from build123d import *

# Parameters (mm, degrees)
F0_W      = 59.0042
F0_H      = 41.021
F1_DEPTH  = 13.97
F2_R      = 2.54
F3_W      = 36.449
F3_H      = 36.449
F4_DEPTH  = 11.43
F5_W      = 25.146
F5_H      = 25.146
F6_DEPTH  = 2.541
F7_R      = 1.5875
F8_DEPTH  = 12.7
F9_W      = 9.144
F9_H      = 13.97
F10_DEPTH = 25.019
F11_R     = 6.98499
F12_W     = 3.3528
F12_H     = 22.225
F13_DEPTH = 13.971
F14_R     = 2.54
F15_DEPTH = 34.0878


# Not quite as in the source:
# - a fillet or chamfer is up to 0.001 mm smaller than in the source, because OpenCascade refuses the exact size


with BuildPart() as f1:
    # F0 (on Top) → F1 (new body)
    with BuildSketch(Plane.XY):
        with Locations((4.1021, 4.8895)):
            Rectangle(F0_W, F0_H)
    extrude(amount=F1_DEPTH)

    # F2
    f2_edges = [f1.edges().sort_by_distance(p)[0] for p in [
        (-25.4, 25.4, 6.985),
        (33.6042, 25.4, 6.985),
        (33.6042, -15.621, 6.985),
        (-25.4, -15.621, 6.985),
    ]]
    fillet(f2_edges, radius=F2_R)

    # F3 (on face) → F4 (cut)
    with BuildSketch(Plane.XY.offset(13.97)):
        with Locations((3.9497, 4.8895)):
            Rectangle(F3_W, F3_H)
    extrude(amount=-F4_DEPTH, mode=Mode.SUBTRACT)

    # F5 (on face) → F6 (cut, through all)
    with BuildSketch(Plane.XY.offset(2.54)):
        with Locations((3.937, 4.9022)):
            Rectangle(F5_W, F5_H)
    extrude(amount=-F6_DEPTH, mode=Mode.SUBTRACT)

    # F7 (on face) → F8 (cut)
    with BuildSketch(Plane.XY.offset(13.97)):
        with Locations((-20.32, 20.32)):
            Circle(F7_R)
        with Locations((-20.32, -10.541)):
            Circle(F7_R)
        with Locations((28.5242, 20.32)):
            Circle(F7_R)
        with Locations((28.5242, -10.541)):
            Circle(F7_R)
    extrude(amount=-F8_DEPTH, mode=Mode.SUBTRACT)

    # F9 (on face) → F10 (join)
    with BuildSketch(Plane(origin=(0, 25.4, 0), x_dir=(-1, 0, 0), z_dir=(0, 1, 0))):
        with Locations((-4.1148, 6.985)):
            Rectangle(F9_W, F9_H)
    extrude(amount=F10_DEPTH)

    # F11 (radius 6.985 in the source; OpenCascade refuses exactly that, so slightly less here)
    f11_edges = [f1.edges().sort_by_distance(p)[0] for p in [
        (4.1148, 50.419, 13.97),
        (4.1148, 50.419, 0),
    ]]
    fillet(f11_edges, radius=F11_R)

    # F12 (on face) → F13 (cut, through all)
    with BuildSketch(Plane.XY.offset(13.97)):
        with Locations((4.1148, 42.8625)):
            Rectangle(F12_W, F12_H)
    extrude(amount=-F13_DEPTH, mode=Mode.SUBTRACT)

    # F14 (on face) → F15 (cut, through all)
    with BuildSketch(Plane.YZ.offset(8.6868)):
        with Locations((43.434, 6.985)):
            Circle(F14_R)
    extrude(amount=-F15_DEPTH, mode=Mode.SUBTRACT)


solid = f1.part
Build history of the part. All positions in model axes, mm. A direction names the side the tool comes from. Coordinates: 2 decimals unless noted, no trailing zeros. Write each loop counter-clockwise with the first axis right and the second up, starting at its lowest first coordinate (ties: lowest second). Pieces come first, ordered by that corner, then holes. Notation, with made-up numbers: (37.5, 18) -> (73.5, 18) arc R22 cw to (73.5, 43) -> close; hole circle Ø6 at (44, -10.75). An arc over 180 degrees is marked (long way). Use CSV: the item, a comma, the result in double quotes. Start each with the question number.
Q1. Pull direction Y, two halves, no side cores. Call faces 4 (the flat face through (4, 17.475, 1)), 5 (the cylindrical face through (0.97, 48.319, 11.978)), 6 (the flat face through (-0.457, 38, 7)): released by +Y, released by -Y, zero draft, split by the parting line, or undercut.
Q2. Flat gauge pins, fed straight in: pin 1 Ø7 at (x, z) = (-13, 7.5) entering from +Y; pin 2 Ø1 at (x, y) = (28, 20.5) entering from +Z; pin 3 Ø6 at (x, y) = (18, 1) entering from +Z; pin 4 Ø10 at (x, y) = (4.5, 12) entering from -Z. Where does each tip first touch, or does it go through?
Q3. Cut at A-A, the plane y = -0.5. List the corners of the cut face in (x, z).
Q4. 3-axis set-ups, long thin cutter, end or side, ignore diameter. For faces 1 (the cylindrical face through (1.011, 45.857, 7.748)), 2 (the flat face through (5.791, 39, 7)), 3 (the flat face through (-14.275, 5, 8)): which of +Z, -Z, +X, -X, +Y, -Y reach the whole face in a straight line?
Q5. Drill centre lines: probe 1 along Y at (x, z) = (-20.32, 9.75); probe 2 along Y at (x, z) = (4, 1.5); probe 3 along Y at (x, z) = (-13.5, 5.5) (3 decimals). Where is each one in solid material? Low to high.
Q6. Cut at B-B, the plane z = 6.25. State how many separate pieces and enclosed holes the cut face has, then the cut area to 3 significant figures.
Q7. Cut at C-C, the plane x = 5. List the corners of the cut face in (y, z) (3 decimals).
Q8. Cut at D-D, the plane y = 20.32. List the corners of the cut face in (x, z).
Checked values:
1,face 4,"undercut"
1,face 5,"released by +Y"
1,face 6,"zero draft"
2,pin 1,"stops at y = 25.4"
2,pin 2,"stops at z = 1.27"
2,pin 3,"stops at z = 2.54"
2,pin 4,"passes through"
3,outline,"(-25.4, 0) -> (-8.64, 0) -> (-8.64, 2.54) -> (-14.27, 2.54) -> (-14.27, 13.97) -> (-25.4, 13.97) -> close; (16.51, 0) -> (33.6, 0) -> (33.6, 13.97) -> (22.17, 13.97) -> (22.17, 2.54) -> (16.51, 2.54) -> close"
4,face 1,"+X, -X"
4,face 2,"+Z, -Z, +Y"
4,face 3,"+Z"
5,probe 1,"y = -15.62 to -12.13, -8.95 to 18.73, 21.91 to 25.4"
5,probe 2,"y = -15.62 to -7.67, 17.48 to 31.75"
5,probe 3,"y = -15.621 to -13.335, 23.114 to 25.4"
6,separate pieces,"3"
6,enclosed holes,"5"
6,area,"1,190 mm²"
7,outline,"(-15.621, 0) -> (-7.671, 0) -> (-7.671, 2.54) -> (-13.335, 2.54) -> (-13.335, 13.97) -> (-15.621, 13.97) -> close; (17.475, 0) -> (31.75, 0) -> (31.75, 13.97) -> (23.114, 13.97) -> (23.114, 2.54) -> (17.475, 2.54) -> close"
8,outline,"(-25.4, 0) -> (33.6, 0) -> (33.6, 13.97) -> (30.11, 13.97) -> (30.11, 1.27) -> (26.94, 1.27) -> (26.94, 13.97) -> (22.17, 13.97) -> (22.17, 2.54) -> (-14.27, 2.54) -> (-14.27, 13.97) -> (-18.73, 13.97) -> (-18.73, 1.27) -> (-21.91, 1.27) -> (-21.91, 13.97) -> (-25.4, 13.97) -> close"
